Model file for the job. Use its own axes, mm. A direction names the side the tool comes from. Give positions to 0.01 mm unless a question says otherwise; leave off trailing zeros. Order: outer loops, then holes, each group sorted by start corner. A loop starts at its lowest first (then second) coordinate and runs counter-clockwise, first axis right, second up. Notation, with made-up numbers: (23, -34) - (69, -34) arc R29 ccw to (69, 0) - close; hole circle Ø10 at (75.5, 43.25). An arc over 180 degrees is marked (long way). Return JSON: item names as keys, results as strings. Group by question number.
from build123d import *

# Parameters (mm, degrees)
EXTRUDE_1_DEPTH = 1
EXTRUDE_2_DEPTH = 0.1
FILLET_1_R      = 0.5
FILLET_2_R      = 0.5


with BuildPart() as part:
    # 草图1 → 凸台-拉伸1 (new body)
    with BuildSketch(Plane.XY):
        Polygon((-5, 0), (-5, 1.5), (-5.5, 2.5), (-5.5, 7.5), (5.5, 7.5), (5.5, -7.5), (-4.5, -7.5), (-4.5, -2.5), (-5.5, -1.5), (-5.5, 0), align=None)
    extrude(amount=EXTRUDE_1_DEPTH)

    # 草图2 → 凸台-拉伸2 (add)
    with BuildSketch(Plane.XY.offset(1)):
        with BuildLine():
            Line((-5.5, 6), (-5.5, 7.5))
            Line((-5.5, 7.5), (5.5, 7.5))
            Line((5.5, 7.5), (5.5, 6))
            ThreePointArc((5.5, 6), (0, 5.5), (-5.5, 6))
        make_face()
    extrude(amount=EXTRUDE_2_DEPTH)

    # 圆角1
    # the kernel refuses this fillet: 0.5 mm, written as the material it adds along each edge
    with BuildSketch(Plane(origin=(0, 36, 1), x_dir=(0.20445847585132765, -0.9788752380423933, 0), z_dir=(0.9788752380423933, 0.20445847585132765, 0))) as fillet_1_piece_1_section:
        with BuildLine():
            CenterArc((30.8, -0.5), FILLET_1_R, 90, 36.869897646)
            Line((30.5, -0.1), (30.5, 0))
            Line((30.5, 0), (30.8, 0))
        make_face()
    fillet_1_piece_1 = revolve(axis=Axis((0, 36, 1), (0, 0, -1)), revolution_arc=23.595601167, mode=Mode.PRIVATE)
    fillet_1_piece_1 = split(fillet_1_piece_1, bisect_by=Plane(origin=(-5.5, 5.358430111, 1.024709668), z_dir=(1, 0, 0)), keep=Keep.TOP, mode=Mode.PRIVATE)
    fillet_1_piece_1 = split(fillet_1_piece_1, bisect_by=Plane(origin=(5.5, 5.358430111, 1.024709668), z_dir=(-1, 0, 0)), keep=Keep.TOP, mode=Mode.PRIVATE)
    add(fillet_1_piece_1)

    # 圆角2
    fillet_2_edges = [part.edges().sort_by_distance(p)[0] for p in [
        (-5.5, 7.5, 0.55),
        (5.5, 7.5, 0.55),
    ]]
    fillet(fillet_2_edges, radius=FILLET_2_R)


solid = part.part
(1) Slice it at B-B (y = 3.75). Give the cut face in (x, z).
(2) Slice it at A-A (z = 0.75). Give the cut face in (x, y), and give its area (3 significant figures).
(3) Drop flat-ended pins along their axis: pin 1 Ø5 at (x, y) = (3, -1) entering from -Z; pin 2 Ø4 at (x, y) = (2.5, -5.5) entering from +Z. Give the stop position or say it passes through.
(4) Pull direction Y, two halves, no side cores. Call faces 1 (the face through (-0.1, 7.5, 0.5)), 2 (the face through (0, 0, 0)), 3 (the face through (-5, 0.7, 0.5)): released by +Y, released by -Y, zero draft, split by the parting line, or undercut.
(5) Drill centre lines: L1, parallel to Z at x = -4.75, y = 0; L2, parallel to X at y = -6.5, z = 0.75; L3, parallel to X at y = 1, z = 0.8. Where is each one in solid material? Low to high.
(6) Slice it at C-C (y = -5.25). Give the cut face in (x, z), and give its area (3 significant figures).
(7) 3-axis set-ups, long thin cutter, end or side, ignore diameter. For faces 4 (the face through (5.5, -0.4, 0.6)), 5 (the face through (-5.246, 1.993, 0.493)), 6 (the face through (-4.5, -5, 0.5)): which of +Z, -Z, +X, -X, +Y, -Y reach the whole face in a straight line?
Result set:
{
 "1": {"outline": "(-5.5, 0) - (5.5, 0) - (5.5, 1) - (-5.5, 1) - close"},
 "2": {"outline": "(-5.5, -1.5) - (-4.5, -2.5) - (-4.5, -7.5) - (5.5, -7.5) - (5.5, 7) arc R0.5 ccw to (5, 7.5) - (-5, 7.5) arc R0.5 ccw to (-5.5, 7) - (-5.5, 2.5) - (-5, 1.5) - (-5, 0) - (-5.5, 0) - close", "area": "158 mm²"},
 "3": {"pin 1": "stops at z = 0", "pin 2": "stops at z = 1"},
 "4": {"face 1": "released by +Y", "face 2": "zero draft", "face 3": "undercut"},
 "5": {"L1": "z = 0 to 1", "L2": "x = -4.5 to 5.5", "L3": "x = -5 to 5.5"},
 "6": {"outline": "(-4.5, 0) - (5.5, 0) - (5.5, 1) - (-4.5, 1) - close", "area": "10.0 mm²"},
 "7": {"face 4": "+Z, -Z, +X, +Y, -Y", "face 5": "+Z, -Z, -X", "face 6": "+Z, -Z, -X, -Y"}
}
